from build123d import *

# Parameters (mm, degrees)
SKETCH_R      = 26.2
SKETCH_R_2    = 16.2
PAD_DEPTH     = 5.5
SKETCH001_R   = 19
SKETCH001_R_2 = 16.2
PAD001_DEPTH  = 1
FILLET_R      = 5


with BuildPart() as part:
    # Sketch → Pad (new body, symmetric)
    with BuildSketch(Plane.XY):
        Circle(SKETCH_R)
        Circle(SKETCH_R_2, mode=Mode.SUBTRACT)
    extrude(amount=PAD_DEPTH, both=True)

    # Sketch001 → Pad001 (new body)
    with BuildSketch(Plane.XY.offset(5.5)):
        Circle(SKETCH001_R)
        Circle(SKETCH001_R_2, mode=Mode.SUBTRACT)
    extrude(amount=PAD001_DEPTH)

    # Fillet
    fillet_edges = [part.edges().sort_by_distance(p)[0] for p in [
        (-26.2, 0, 5.5),
    ]]
    fillet(fillet_edges, radius=FILLET_R)


solid = part.part
Verification items for the finished model (mm, model axes). A direction names the side the tool comes from. Round coordinates to 2 decimals unless told otherwise and drop trailing zeros. Order: outer loops, then holes, each group sorted by start corner. A loop starts at its lowest first (then second) coordinate and runs counter-clockwise, first axis right, second up. Notation, with made-up numbers: (49, -17.75) -> (81, -17.75) arc R13 cw to (81, -5.75) -> close; hole circle Ø2 at (35.5, -26). An arc over 180 degrees is marked (long way). Put each result on its own line as item: value.
1) Mould release check, pull along Y, two halves, no side actions. Record for faces 1 (the cylindrical face through (-3.512, -15.815, 0.416)), 2 (the cylindrical face through (-3.411, 25.977, -2.458)), 3 (the flat face through (14, 9, 6.5)): +Y half, -Y half, draft (parallel to the pull), parting line (faces both ways), or undercut.
Final values:
face 1: undercut
face 2: parting line
face 3: draft
2) Section check A-A (y = 0). Record the cut outline in (x, z), then the cut area to 3 significant figures.
Final values:
outline: (-26.2, -5.5) -> (-16.2, -5.5) -> (-16.2, 6.5) -> (-19, 6.5) -> (-19, 5.5) -> (-21.2, 5.5) arc R5 ccw to (-26.2, 0.5) -> close; (16.2, -5.5) -> (26.2, -5.5) -> (26.2, 0.5) arc R5 ccw to (21.2, 5.5) -> (19, 5.5) -> (19, 6.5) -> (16.2, 6.5) -> close
area: 215 mm^2
3) Material ranges on line 1 (Y direction, x = 0, z = 0.25); line 2 (X direction, y = 12, z = -0.5), recorded low to high.
Final values:
line 1: y = -26.2 to -16.2, 16.2 to 26.2
line 2: x = -23.29 to -10.88, 10.88 to 23.29
4) Section check C-C (z = -1.5). Record the cut outline in (x, y).
Final values:
outline: circle Ø52.4 at (0, 0); hole circle Ø32.4 at (0, 0)
5) Section check D-D (z = 4). Record the cut outline in (x, y).
Final values:
outline: circle Ø49.54 at (0, 0); hole circle Ø32.4 at (0, 0)
6) Set-up check for faces 4 (the flat face through (-12, -11.3, -5.5)), 5 (the cylindrical face through (8.767, -16.856, 5.993)): record each of +Z, -Z, +X, -X, +Y, -Y from which the full face is reachable in a straight line by a thin tool's end or side.
Final values:
face 4: -Z, +X, -X, +Y, -Y
face 5: +Z
7) Depth check by flat-ended pin: pin 1 (2 mm diameter, centred on x = 18.5, z = 0.5, fed in from -Y); pin 2 (1 mm diameter, centred on y = 1, z = -3, fed in from -X); pin 3 (2 mm diameter, centred on x = 20.5, z = 4, fed in from -Y). Enter the tip coordinate at first touch or a pass-through.
Final values:
pin 1: stops at y = -19.5
pin 2: stops at x = -26.2
pin 3: stops at y = -15.84
